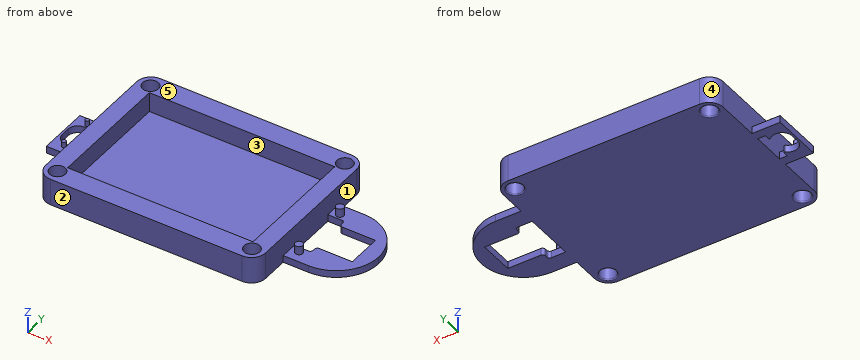
```python
from build123d import *

# Parameters (mm, degrees)
SKETCH1_W               = 55.88
SKETCH1_H               = 83.566
BOSS_EXTRUDE1_DEPTH     = 3.175
SKETCH2_W               = 74.93
SKETCH2_H               = 102.616
SKETCH2_W_2             = 55.88
SKETCH2_H_2             = 83.566
BOSS_EXTRUDE2_DEPTH     = 12.065
CUT_EXTRUDE1_DEPTH      = 65.666075449
CUT_EXTRUDE1_DEPTH_BACK = 65.666075449
SKETCH3_R               = 3.556
CUT_EXTRUDE2_DEPTH      = 65.666075449
CUT_EXTRUDE2_DEPTH_BACK = 65.666075449
SKETCH4_W               = 1.778
SKETCH4_H               = 74.93
FILLET1_R               = 6.35
FILLET2_R               = 0.508
SKETCH5_W               = 38.1
SKETCH5_H               = 3.175
BOSS_EXTRUDE3_DEPTH     = 30.48
CUT_EXTRUDE3_DEPTH      = 89.793346738
CUT_EXTRUDE3_DEPTH_BACK = 89.793346738
SKETCH6_W               = 7.62
SKETCH6_H               = 22.86
SKETCH7_R               = 1.7145
BOSS_EXTRUDE4_DEPTH     = 3.81
CUT_EXTRUDE4_DEPTH      = 89.793346738
CUT_EXTRUDE4_DEPTH_BACK = 89.793346738
SKETCH8_W               = 22.86
SKETCH8_H               = 15.875
SKETCH9_W               = 6.6929
SKETCH9_H               = 15.875
BOSS_EXTRUDE5_DEPTH     = 3.175
FILLET3_R               = 19.05
FILLET5_R               = 1.27
SKETCH10_W              = 22.86
SKETCH10_H              = 3.175
BOSS_EXTRUDE6_DEPTH     = 12.7
CUT_EXTRUDE5_DEPTH      = 89.793346738
CUT_EXTRUDE5_DEPTH_BACK = 89.793346738
SKETCH11_W              = 3.4036
SKETCH11_H              = 14.9352
CUT_EXTRUDE6_DEPTH      = 90.167205575
CUT_EXTRUDE6_DEPTH_BACK = 90.167205575
FILLET7_R               = 0.508
SKETCH13_R              = 0.889
BOSS_EXTRUDE7_DEPTH     = 2.54


with BuildPart() as part:
    # Sketch1 → Boss-Extrude1 (new body)
    with BuildSketch(Plane(origin=(0, 0, 0), x_dir=(0, 1, 0), z_dir=(0, 0, 1))):
        Rectangle(SKETCH1_W, SKETCH1_H)
    extrude(amount=BOSS_EXTRUDE1_DEPTH)

    # Sketch2 → Boss-Extrude2 (add)
    with BuildSketch(Plane(origin=(0, 0, 0), x_dir=(0, 1, 0), z_dir=(0, 0, 1))):
        Rectangle(SKETCH2_W, SKETCH2_H)
        Rectangle(SKETCH2_W_2, SKETCH2_H_2, mode=Mode.SUBTRACT)
    extrude(amount=BOSS_EXTRUDE2_DEPTH)

    # Sketch3 → Cut-Extrude1 (cut, two sides: drawn at the far end of the back side and taken through both)
    with BuildSketch(Plane.XY.offset(12.065).offset(-CUT_EXTRUDE1_DEPTH_BACK)):
        with Locations((-43.815, 31.75)):
            Circle(SKETCH3_R)
        with Locations((43.815, 31.75)):
            Circle(SKETCH3_R)
        with Locations((43.815, -31.75)):
            Circle(SKETCH3_R)
        with Locations((-43.815, -31.75)):
            Circle(SKETCH3_R)
    extrude(amount=CUT_EXTRUDE1_DEPTH + CUT_EXTRUDE1_DEPTH_BACK, mode=Mode.SUBTRACT)

    # Sketch4 → Cut-Extrude2 (cut, two sides: drawn at the far end of the back side and taken through both)
    with BuildSketch(Plane.XY.offset(12.065).offset(-CUT_EXTRUDE2_DEPTH_BACK)):
        with Locations((-50.419, 0)):
            Rectangle(SKETCH4_W, SKETCH4_H)
        with Locations((50.419, 0)):
            Rectangle(SKETCH4_W, SKETCH4_H)
    extrude(amount=CUT_EXTRUDE2_DEPTH + CUT_EXTRUDE2_DEPTH_BACK, mode=Mode.SUBTRACT)

    # Fillet1
    fillet1_edges = [part.edges().sort_by_distance(p)[0] for p in [
        (-49.53, -37.465, 6.0325),
        (-49.53, 37.465, 6.0325),
        (49.53, 37.465, 6.0325),
        (49.53, -37.465, 6.0325),
    ]]
    fillet(fillet1_edges, radius=FILLET1_R)

    # Fillet2
    fillet2_edges = [part.edges().sort_by_distance(p)[0] for p in [
        (-47.371, -31.75, 0),
        (40.259, -31.75, 0),
        (40.259, 31.75, 0),
        (-47.371, 31.75, 0),
    ]]
    fillet(fillet2_edges, radius=FILLET2_R)

    # Sketch5 → Boss-Extrude3 (add)
    with BuildSketch(Plane.YZ.offset(49.53)):
        with Locations((0, 1.5875)):
            Rectangle(SKETCH5_W, SKETCH5_H)
    extrude(amount=BOSS_EXTRUDE3_DEPTH)

    # Sketch6 → Cut-Extrude3 (cut, two sides: drawn at the far end of the back side and taken through both)
    with BuildSketch(Plane.XY.offset(3.175).offset(-CUT_EXTRUDE3_DEPTH_BACK)):
        with Locations((53.34, 0)):
            Rectangle(SKETCH6_W, SKETCH6_H)
    extrude(amount=CUT_EXTRUDE3_DEPTH + CUT_EXTRUDE3_DEPTH_BACK, mode=Mode.SUBTRACT)

    # Sketch7 → Boss-Extrude4 (add)
    with BuildSketch(Plane.XY.offset(3.175)):
        with Locations(Location((53.3019, 13.9573, 0), (0, 0, 180))):
            Circle(SKETCH7_R)
        with Locations(Location((53.3019, -13.9573, 0), (0, 0, 180))):
            Circle(SKETCH7_R)
    extrude(amount=BOSS_EXTRUDE4_DEPTH)

    # Sketch8 → Cut-Extrude4 (cut, two sides: drawn at the far end of the back side and taken through both)
    with BuildSketch(Plane.XY.offset(3.175).offset(-CUT_EXTRUDE4_DEPTH_BACK)):
        with Locations((68.58, 0)):
            Rectangle(SKETCH8_W, SKETCH8_H)
    extrude(amount=CUT_EXTRUDE4_DEPTH + CUT_EXTRUDE4_DEPTH_BACK, mode=Mode.SUBTRACT)

    # Sketch9 → Boss-Extrude5 (add)
    with BuildSketch(Plane.XY.offset(3.175)):
        with Locations((76.66355, 0)):
            Rectangle(SKETCH9_W, SKETCH9_H)
    extrude(amount=-BOSS_EXTRUDE5_DEPTH)

    # Fillet3
    fillet3_edges = [part.edges().sort_by_distance(p)[0] for p in [
        (80.01, -19.05, 1.5875),
        (80.01, 19.05, 1.5875),
    ]]
    fillet(fillet3_edges, radius=FILLET3_R - 0.0001)  # a hair under: the kernel refuses the full size

    # Fillet5
    fillet5_edges = [part.edges().sort_by_distance(p)[0] for p in [
        (57.15, 11.43, 1.5875),
        (57.15, -11.43, 1.5875),
        (57.15, 7.9375, 1.5875),
        (57.15, -7.9375, 1.5875),
    ]]
    fillet(fillet5_edges, radius=FILLET5_R)

    # Sketch10 → Boss-Extrude6 (add)
    with BuildSketch(Plane(origin=(-49.53, 0, 0), x_dir=(0, -1, 0), z_dir=(-1, 0, 0))):
        with Locations((0, 1.5875)):
            Rectangle(SKETCH10_W, SKETCH10_H)
    extrude(amount=BOSS_EXTRUDE6_DEPTH)

    # Sketch11 → Cut-Extrude5 (cut, two sides: drawn at the far end of the back side and taken through both)
    with BuildSketch(Plane.XY.offset(3.175).offset(-CUT_EXTRUDE5_DEPTH_BACK)):
        with Locations((-51.2318, 0)):
            Rectangle(SKETCH11_W, SKETCH11_H)
    extrude(amount=CUT_EXTRUDE5_DEPTH + CUT_EXTRUDE5_DEPTH_BACK, mode=Mode.SUBTRACT)

    # Sketch12 → Cut-Extrude6 (cut, two sides: drawn at the far end of the back side and taken through both)
    with BuildSketch(Plane(origin=(0, 0, 0), x_dir=(1, 0, 0), z_dir=(0, 0, -1)).offset(-CUT_EXTRUDE6_DEPTH_BACK)):
        with BuildLine():
            Line((-52.451, 1.905), (-52.451, -1.905))
            ThreePointArc((-52.451, -1.905), (-56.896, -6.35), (-61.341, -1.905))
            Line((-61.341, -1.905), (-61.341, 1.905))
            ThreePointArc((-61.341, 1.905), (-56.896, 6.35), (-52.451, 1.905))
        make_face()
    extrude(amount=CUT_EXTRUDE6_DEPTH + CUT_EXTRUDE6_DEPTH_BACK, mode=Mode.SUBTRACT)

    # Fillet7
    fillet7_edges = [part.edges().sort_by_distance(p)[0] for p in [
        (-52.9336, 3.919301676, 1.5875),
        (-52.9336, -3.919301676, 1.5875),
    ]]
    fillet(fillet7_edges, radius=FILLET7_R)

    # Sketch13 → Boss-Extrude7 (add)
    with BuildSketch(Plane.XY.offset(3.175)):
        with Locations(Location((-56.642, 7.8994, 0), (0, 0, 90))):
            Circle(SKETCH13_R)
        with Locations(Location((-56.642, -7.8994, 0), (0, 0, 90))):
            Circle(SKETCH13_R)
    extrude(amount=BOSS_EXTRUDE7_DEPTH)


solid = part.part
```
The model under review builds one solid part; all positions refer to its coordinate system, in mm. Face numbers are marked on the shaded views. A direction names the side the tool comes from. Round coordinates to 2 decimals unless told otherwise and drop trailing zeros. Order: outer loops, then holes, each group sorted by start corner. A loop starts at its lowest first (then second) coordinate and runs counter-clockwise, first axis right, second up. Notation, with made-up numbers: (-29, 10.25) -> (7, 10.25) arc R24 ccw to (7, 49.25) -> close; hole circle Ø10 at (-9, 23.5). An arc over 180 degrees is marked (long way). Use a Markdown table: item, result.
Q1. We need section B-B on x = 64.5. Write out the cut boundary in (y, z) (1 decimal).
Values:
| item | result |
|---|---|
| outline | (-18.7, 0) -> (-7.9, 0) -> (-7.9, 3.2) -> (-18.7, 3.2) -> close; (7.9, 0) -> (18.7, 0) -> (18.7, 3.2) -> (7.9, 3.2) -> close |
Q2. We need section D-D on x = 24.5. Write out the cut boundary in (y, z) (3 decimals).
Values:
| item | result |
|---|---|
| outline | (-37.465, 0) -> (37.465, 0) -> (37.465, 12.065) -> (27.94, 12.065) -> (27.94, 3.175) -> (-27.94, 3.175) -> (-27.94, 12.065) -> (-37.465, 12.065) -> close |
Q3. We need section C-C on y = -22.5. Write out the cut boundary in (x, z) (3 decimals), then the cut area to 3 significant figures.
Values:
| item | result |
|---|---|
| outline | (-49.53, 0) -> (49.53, 0) -> (49.53, 12.065) -> (41.783, 12.065) -> (41.783, 3.175) -> (-41.783, 3.175) -> (-41.783, 12.065) -> (-49.53, 12.065) -> close |
| area | 452 mm^2 |
Q4. Mouldability with a two-part tool opening along X and no side actions: class the marked faces 3, 4 and 5 as +X half, -X half, draft (parallel to the pull), parting line (faces both ways), or undercut.
Values:
| item | result |
|---|---|
| face 3 | undercut |
| face 4 | -X half |
| face 5 | draft |
Q5. Tool access review of the marked faces 1 and 2: name each direction out of +Z, -Z, +X, -X, +Y, -Y from which nothing blocks a thin tool from reaching the whole face with its end or side.
Values:
| item | result |
|---|---|
| face 1 | +Z |
| face 2 | +Z, -Z, +X, -X, -Y |
Q6. We need section A-A on z = 8.5. Write out the cut boundary in (x, y) (3 decimals), then the cut area to 3 significant figures.
Values:
| item | result |
|---|---|
| outline | (-49.53, -31.115) arc R6.35 ccw to (-43.18, -37.465) -> (43.18, -37.465) arc R6.35 ccw to (49.53, -31.115) -> (49.53, 31.115) arc R6.35 ccw to (43.18, 37.465) -> (-43.18, 37.465) arc R6.35 ccw to (-49.53, 31.115) -> close; hole circle Ø7.112 at (-43.815, -31.75); hole circle Ø7.112 at (-43.815, 31.75); hole (-41.783, -27.94) -> (41.783, -27.94) -> (41.783, 27.94) -> (-41.783, 27.94) -> close; hole circle Ø7.112 at (43.815, -31.75); hole circle Ø7.112 at (43.815, 31.75) |
| area | 2,560 mm^2 |
Q7. For line 1 (X direction, y = -31.75, z = 7); line 2 (Y direction, x = 18, z = 6.75) (3 decimals); line 3 (X direction, y = 1, z = 8.25), list the stretches that pass through material, from the lowest coordinate up.
Values:
| item | result |
|---|---|
| line 1 | x = -49.5 to -47.37, -40.26 to 40.26, 47.37 to 49.5 |
| line 2 | y = -37.465 to -27.94, 27.94 to 37.465 |
| line 3 | x = -49.53 to -41.78, 41.78 to 49.53 |
Q8. Clearance check with flat-ended pins moving along their axes: P1, Ø2, axis at y = -6, z = 1.5, coming from the +X side; P2, Ø1.6, axis at x = -58.5, z = 1.5, coming from the -Y side; P3, Ø2, axis at y = 6.5, z = 1, coming from the +X side. State where each tip first meets the part, or that it passes through.
Values:
| item | result |
|---|---|
| P1 | stops at x = 79.34 |
| P2 | stops at y = -11.43 |
| P3 | stops at x = 79.2 |
